```python
from build123d import *
from OCP.BRepFilletAPI import BRepFilletAPI_MakeChamfer

# Parameters (mm, degrees)
SKETCH_1_W               = 23
SKETCH_1_H               = 90
EXTRUDE_1_DEPTH          = 5
SKETCH_2_R               = 4.25
SKETCH_2_R_2             = 6.5
CUT_EXTRUDE_1_DEPTH      = 3.5
EXTRUDE_START            = 15
SKETCH_4_W               = 5
SKETCH_4_H               = 13
EXTRUDE_3_DEPTH          = 30
FILLET_2_R               = 10
CUT_EXTRUDE_2_DEPTH      = 50.812147113
CUT_EXTRUDE_2_DEPTH_BACK = 50.812147113
SKETCH_5_R               = 1.75
FILLET_3_R               = 2.5
EXTRUDE_START_2          = 6.5
EXTRUDE_4_DEPTH          = 5
CHAMFER_1_SIZE           = 1.2
CHAMFER_1_SIZE2          = 0.692820323
FILLET_4_R               = 3


with BuildPart() as part:
    # 스케치1 → 보스-돌출1 (new, symmetric)
    with BuildSketch(Plane(origin=(0, 0, 0), x_dir=(1, 0, 0), z_dir=(0, 1, 0))):
        Rectangle(SKETCH_1_W, SKETCH_1_H)
    extrude(amount=EXTRUDE_1_DEPTH, both=True)

    # 스케치2 → 컷-돌출1 (cut)
    with BuildSketch(Plane.XZ.offset(5)):
        with Locations((0, 24.25)):
            Circle(SKETCH_2_R)
        with BuildLine():
            ThreePointArc((4.25, 24.25), (-0.19737792, 20.004585773), (-4.231666803, 24.644329897))
            Line((-4.231666803, 24.644329897), (-6.471960993, 0.603092784))
            ThreePointArc((-6.471960993, 0.603092784), (0, 6.5), (6.471960993, 0.603092784))
            Line((6.471960993, 0.603092784), (4.231666803, 24.644329897))
            ThreePointArc((4.231666803, 24.644329897), (4.245414227, 24.44737792), (4.25, 24.25))
        make_face()
        Circle(SKETCH_2_R_2)
        with BuildLine():
            ThreePointArc((6.471960993, -0.603092784), (0, -6.5), (-6.471960993, -0.603092784))
            Line((-6.471960993, -0.603092784), (-4.231666803, -24.644329897))
            ThreePointArc((-4.231666803, -24.644329897), (-0.19737792, -20.004585773), (4.25, -24.25))
            ThreePointArc((4.25, -24.25), (4.245414227, -24.44737792), (4.231666803, -24.644329897))
            Line((4.231666803, -24.644329897), (6.471960993, -0.603092784))
        make_face()
        with Locations((0, -24.25)):
            Circle(SKETCH_2_R)
    extrude(amount=-CUT_EXTRUDE_1_DEPTH, mode=Mode.SUBTRACT)

    # 스케치4 → 보스-돌출3 (add)
    with BuildSketch(Plane.XY.offset(EXTRUDE_START)):
        with Locations((-9, 11.5)):
            Rectangle(SKETCH_4_W, SKETCH_4_H)
        with Locations((9, 11.5)):
            Rectangle(SKETCH_4_W, SKETCH_4_H)
    extrude(amount=EXTRUDE_3_DEPTH)

    # 필렛2
    fillet_2_edges = [part.edges().sort_by_distance(p)[0] for p in [
        (-11.5, 0, -45),
        (11.5, 0, -45),
    ]]
    fillet(fillet_2_edges, radius=FILLET_2_R)

    # 스케치5 → 컷-돌출2 (cut, two sides: drawn at the far end of the back side and taken through both)
    with BuildSketch(Plane(origin=(0, 0, 0), x_dir=(0, 0, -1), z_dir=(1, 0, 0)).offset(-CUT_EXTRUDE_2_DEPTH_BACK)):
        with Locations((-22.5, 11.5)):
            Circle(SKETCH_5_R)
        with Locations((-37.5, 11.5)):
            Circle(SKETCH_5_R)
    extrude(amount=CUT_EXTRUDE_2_DEPTH + CUT_EXTRUDE_2_DEPTH_BACK, mode=Mode.SUBTRACT)

    # 필렛3
    fillet_3_edges = [part.edges().sort_by_distance(p)[0] for p in [
        (11.5, 6.5, 45),
        (-11.5, 6.5, 45),
    ]]
    fillet(fillet_3_edges, radius=FILLET_3_R)

    # 스케치6 → 보스-돌출4 (add)
    with BuildSketch(Plane(origin=(0, 0, 0), x_dir=(0, 0, -1), z_dir=(1, 0, 0)).offset(EXTRUDE_START_2)):
        Polygon((-15, 18), (25, 5), (-15, 5), align=None)
    extrude_4 = extrude(amount=EXTRUDE_4_DEPTH)

    # 대칭 복사1: 보스-돌출4 across plane
    add(extrude_4.mirror(Plane(origin=(0, 0, 0), x_dir=(0, 0, 1), z_dir=(1, 0, 0))))

    # 모따기1: one chamfer whose edges measure the first distance from different faces: ONE call of the kernel's chamfer builder (chamfer() names one face for all edges)
    chamfer_1_edges_1 = [part.edges().sort_by_distance(p)[0] for p in [
        (5.351813898, -5, 12.62371134),
    ]]
    chamfer_1_side_1 = [part.faces().sort_by_distance(p)[0] for p in [
        (5.351813898, -3.25, 12.62371134),
    ]]
    chamfer_1_edges_2 = [part.edges().sort_by_distance(p)[0] for p in [
        (5.351813898, -5, -12.62371134),
    ]]
    chamfer_1_side_2 = [part.faces().sort_by_distance(p)[0] for p in [
        (5.351813898, -3.25, -12.62371134),
    ]]
    chamfer_1_edges_3 = [part.edges().sort_by_distance(p)[0] for p in [
        (0, -5, 28.5),
    ]]
    chamfer_1_side_3 = [part.faces().sort_by_distance(p)[0] for p in [
        (0, -3.25, 28.5),
    ]]
    chamfer_1_edges_4 = [part.edges().sort_by_distance(p)[0] for p in [
        (-5.351813898, -5, 12.62371134),
    ]]
    chamfer_1_side_4 = [part.faces().sort_by_distance(p)[0] for p in [
        (-5.351813898, -3.25, 12.62371134),
    ]]
    chamfer_1_edges_5 = [part.edges().sort_by_distance(p)[0] for p in [
        (-6.5, -5, 0),
    ]]
    chamfer_1_side_5 = [part.faces().sort_by_distance(p)[0] for p in [
        (-6.5, -3.25, 0),
    ]]
    chamfer_1_edges_6 = [part.edges().sort_by_distance(p)[0] for p in [
        (-5.351813898, -5, -12.62371134),
    ]]
    chamfer_1_side_6 = [part.faces().sort_by_distance(p)[0] for p in [
        (-5.351813898, -3.25, -12.62371134),
    ]]
    chamfer_1_edges_7 = [part.edges().sort_by_distance(p)[0] for p in [
        (0, -5, -28.5),
    ]]
    chamfer_1_side_7 = [part.faces().sort_by_distance(p)[0] for p in [
        (0, -3.25, -28.5),
    ]]
    chamfer_1_edges_8 = [part.edges().sort_by_distance(p)[0] for p in [
        (6.5, -5, 0),
    ]]
    chamfer_1_side_8 = [part.faces().sort_by_distance(p)[0] for p in [
        (6.5, -3.25, 0),
    ]]
    chamfer_1_edges_9 = [part.edges().sort_by_distance(p)[0] for p in [
        (0, -5, -45),
    ]]
    chamfer_1_side_9 = [part.faces().sort_by_distance(p)[0] for p in [
        (0, 0, -45),
    ]]
    chamfer_1_edges_10 = [part.edges().sort_by_distance(p)[0] for p in [
        (-11.5, -5, 3.75),
    ]]
    chamfer_1_side_10 = [part.faces().sort_by_distance(p)[0] for p in [
        (-11.5, 4.599741569, 9.495989177),
    ]]
    chamfer_1_edges_11 = [part.edges().sort_by_distance(p)[0] for p in [
        (-8.571067812, -5, -42.071067812),
    ]]
    chamfer_1_side_11 = [part.faces().sort_by_distance(p)[0] for p in [
        (-8.571067812, 0, -42.071067812),
    ]]
    chamfer_1_edges_12 = [part.edges().sort_by_distance(p)[0] for p in [
        (8.571067812, -5, -42.071067812),
    ]]
    chamfer_1_side_12 = [part.faces().sort_by_distance(p)[0] for p in [
        (8.571067812, 0, -42.071067812),
    ]]
    chamfer_1_edges_13 = [part.edges().sort_by_distance(p)[0] for p in [
        (0, -5, 45),
    ]]
    chamfer_1_side_13 = [part.faces().sort_by_distance(p)[0] for p in [
        (0, 3.051020408, 45),
    ]]
    chamfer_1_edges_14 = [part.edges().sort_by_distance(p)[0] for p in [
        (11.5, -5, 3.75),
    ]]
    chamfer_1_side_14 = [part.faces().sort_by_distance(p)[0] for p in [
        (11.5, 4.599741569, 9.495989177),
    ]]
    chamfer_1_edges_15 = [part.edges().sort_by_distance(p)[0] for p in [
        (10.767766953, -5, 44.267766953),
    ]]
    chamfer_1_side_15 = [part.faces().sort_by_distance(p)[0] for p in [
        (10.767766953, 6.5, 44.267766953),
    ]]
    chamfer_1_edges_16 = [part.edges().sort_by_distance(p)[0] for p in [
        (-10.767766953, -5, 44.267766953),
    ]]
    chamfer_1_side_16 = [part.faces().sort_by_distance(p)[0] for p in [
        (-10.767766953, 6.5, 44.267766953),
    ]]
    chamfer_1 = BRepFilletAPI_MakeChamfer(part.part.solid().wrapped)
    for e in chamfer_1_edges_1:
        chamfer_1.Add(CHAMFER_1_SIZE, CHAMFER_1_SIZE2, e.wrapped, chamfer_1_side_1[0].wrapped)  # the first distance lies on this face
    for e in chamfer_1_edges_2:
        chamfer_1.Add(CHAMFER_1_SIZE, CHAMFER_1_SIZE2, e.wrapped, chamfer_1_side_2[0].wrapped)  # the first distance lies on this face
    for e in chamfer_1_edges_3:
        chamfer_1.Add(CHAMFER_1_SIZE, CHAMFER_1_SIZE2, e.wrapped, chamfer_1_side_3[0].wrapped)  # the first distance lies on this face
    for e in chamfer_1_edges_4:
        chamfer_1.Add(CHAMFER_1_SIZE, CHAMFER_1_SIZE2, e.wrapped, chamfer_1_side_4[0].wrapped)  # the first distance lies on this face
    for e in chamfer_1_edges_5:
        chamfer_1.Add(CHAMFER_1_SIZE, CHAMFER_1_SIZE2, e.wrapped, chamfer_1_side_5[0].wrapped)  # the first distance lies on this face
    for e in chamfer_1_edges_6:
        chamfer_1.Add(CHAMFER_1_SIZE, CHAMFER_1_SIZE2, e.wrapped, chamfer_1_side_6[0].wrapped)  # the first distance lies on this face
    for e in chamfer_1_edges_7:
        chamfer_1.Add(CHAMFER_1_SIZE, CHAMFER_1_SIZE2, e.wrapped, chamfer_1_side_7[0].wrapped)  # the first distance lies on this face
    for e in chamfer_1_edges_8:
        chamfer_1.Add(CHAMFER_1_SIZE, CHAMFER_1_SIZE2, e.wrapped, chamfer_1_side_8[0].wrapped)  # the first distance lies on this face
    for e in chamfer_1_edges_9:
        chamfer_1.Add(CHAMFER_1_SIZE, CHAMFER_1_SIZE2, e.wrapped, chamfer_1_side_9[0].wrapped)  # the first distance lies on this face
    for e in chamfer_1_edges_10:
        chamfer_1.Add(CHAMFER_1_SIZE, CHAMFER_1_SIZE2, e.wrapped, chamfer_1_side_10[0].wrapped)  # the first distance lies on this face
    for e in chamfer_1_edges_11:
        chamfer_1.Add(CHAMFER_1_SIZE, CHAMFER_1_SIZE2, e.wrapped, chamfer_1_side_11[0].wrapped)  # the first distance lies on this face
    for e in chamfer_1_edges_12:
        chamfer_1.Add(CHAMFER_1_SIZE, CHAMFER_1_SIZE2, e.wrapped, chamfer_1_side_12[0].wrapped)  # the first distance lies on this face
    for e in chamfer_1_edges_13:
        chamfer_1.Add(CHAMFER_1_SIZE, CHAMFER_1_SIZE2, e.wrapped, chamfer_1_side_13[0].wrapped)  # the first distance lies on this face
    for e in chamfer_1_edges_14:
        chamfer_1.Add(CHAMFER_1_SIZE, CHAMFER_1_SIZE2, e.wrapped, chamfer_1_side_14[0].wrapped)  # the first distance lies on this face
    for e in chamfer_1_edges_15:
        chamfer_1.Add(CHAMFER_1_SIZE, CHAMFER_1_SIZE2, e.wrapped, chamfer_1_side_15[0].wrapped)  # the first distance lies on this face
    for e in chamfer_1_edges_16:
        chamfer_1.Add(CHAMFER_1_SIZE, CHAMFER_1_SIZE2, e.wrapped, chamfer_1_side_16[0].wrapped)  # the first distance lies on this face
    add(Compound.cast(chamfer_1.Shape()), mode=Mode.REPLACE)

    # 필렛4
    fillet_4_edges = [part.edges().sort_by_distance(p)[0] for p in [
        (5.351813898, -3.8, -12.62371134),
        (6.5, -3.8, 0),
        (0, -3.8, -28.5),
        (5.351813898, -3.8, 12.62371134),
        (-5.351813898, -3.8, -12.62371134),
        (0, -3.8, 28.5),
        (-6.5, -3.8, 0),
        (-5.351813898, -3.8, 12.62371134),
        (-11.5, -3.8, 3.75),
        (-10.767766953, -3.8, 44.267766953),
        (-8.571067812, -3.8, -42.071067812),
        (0, -3.8, 45),
        (0, -3.8, -45),
        (10.767766953, -3.8, 44.267766953),
        (8.571067812, -3.8, -42.071067812),
        (11.5, -3.8, 3.75),
    ]]
    fillet(fillet_4_edges, radius=FILLET_4_R)


solid = part.part
```
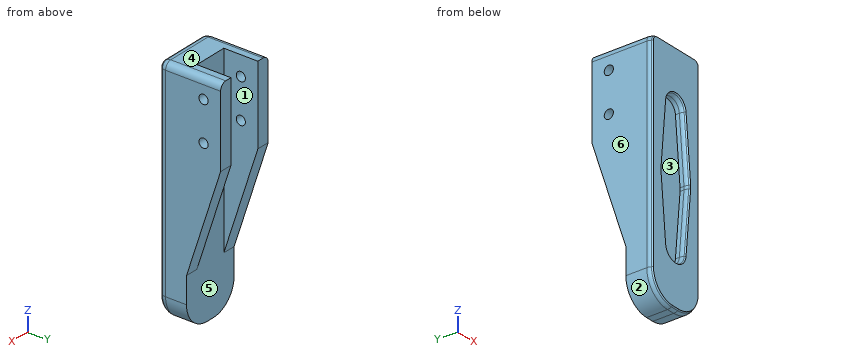
Input: part model. Units: mm. Frame: model coordinates. Face numbers are marked on the shaded views. A direction names the side the tool comes from. Round coordinates to 2 decimals unless told otherwise and drop trailing zeros. Order: outer loops, then holes, each group sorted by start corner. A loop starts at its lowest first (then second) coordinate and runs counter-clockwise, first axis right, second up. Notation, with made-up numbers: (-20.5, 9.25) - (6.5, 9.25) arc R12 ccw to (6.5, 15.25) - close; hole circle Ø1 at (-30, -15). An arc over 180 degrees is marked (long way). Answer in a Markdown table with one row per item.
Item 1: Reachability of the marked faces 1 and 2 from +Z, -Z, +X, -X, +Y, -Y: full face, straight path, thin tool, end or side. Return the list, or none.
Model answer:
| item | result |
|---|---|
| face 1 | +Z, -Z, +Y |
| face 2 | -Z, -X, +Y, -Y |
Item 2: Section query B-B (z = 37.5). Return the cut outline in (x, y).
Model answer:
| item | result |
|---|---|
| outline | (-11.5, -3) arc R3 ccw to (-11.1, -4.5) - (-10.81, -5) - (10.81, -5) - (11.1, -4.5) arc R3 ccw to (11.5, -3) - (11.5, 9.75) - (6.5, 9.75) - (6.5, 5) - (-6.5, 5) - (-6.5, 9.75) - (-11.5, 9.75) - close; (-11.5, 13.25) - (-6.5, 13.25) - (-6.5, 18) - (-11.5, 18) - close; (6.5, 13.25) - (11.5, 13.25) - (11.5, 18) - (6.5, 18) - close |
Item 3: Mould query, pull axis X, two halves, no side actions, for the marked faces 3, 4, 5 and 6. Classes: released by +X, released by -X, zero draft, split by the parting line, or undercut.
Model answer:
| item | result |
|---|---|
| face 3 | undercut |
| face 4 | zero draft |
| face 5 | undercut |
| face 6 | released by -X |
Item 4: Line query: line 1 (X direction, y = 11, z = 17.5); line 2 (Y direction, x = 10.5, z = 37.5); line 3 (Y direction, x = -6.25, z = 39). Output: solid intervals per line, ascending.
Model answer:
| item | result |
|---|---|
| line 1 | x = -11.5 to -6.5, 6.5 to 11.5 |
| line 2 | y = -5 to 9.75, 13.25 to 18 |
| line 3 | y = -5 to 5 |
Item 5: Section query C-C (y = 15). Return the cut outline in (x, z).
Model answer:
| item | result |
|---|---|
| outline | (-11.5, 5.77) - (-6.5, 5.77) - (-6.5, 45) - (-9, 45) arc R2.5 ccw to (-11.5, 42.5) - close; (6.5, 5.77) - (11.5, 5.77) - (11.5, 42.5) arc R2.5 ccw to (9, 45) - (6.5, 45) - close |
Item 6: Section query A-A (y = 11.5). Return the cut outline in (x, z), then the cut area to 3 significant figures.
Model answer:
| item | result |
|---|---|
| outline | (-11.5, -5) - (-6.5, -5) - (-6.5, 20.75) - (-11.5, 20.75) - close; (-11.5, 24.25) - (-6.5, 24.25) - (-6.5, 35.75) - (-11.5, 35.75) - close; (-11.5, 39.25) - (-6.5, 39.25) - (-6.5, 45) - (-9, 45) arc R2.5 ccw to (-11.5, 42.5) - close; (6.5, -5) - (11.5, -5) - (11.5, 20.75) - (6.5, 20.75) - close; (6.5, 24.25) - (11.5, 24.25) - (11.5, 35.75) - (6.5, 35.75) - close; (6.5, 39.25) - (11.5, 39.25) - (11.5, 42.5) arc R2.5 ccw to (9, 45) - (6.5, 45) - close |
| area | 427 mm² |
Item 7: Section query D-D (y = 3). Return the cut outline in (x, z), then the cut area to 3 significant figures.
Model answer:
| item | result |
|---|---|
| outline | (-11.5, -35) arc R10 ccw to (-1.5, -45) - (1.5, -45) arc R10 ccw to (11.5, -35) - (11.5, 42.5) arc R2.5 ccw to (9, 45) - (-9, 45) arc R2.5 ccw to (-11.5, 42.5) - close |
| area | 2,020 mm² |
Item 8: Pin query (flat end, axial travel): pin 1 (2 mm diameter, centred on x = 4.5, y = 14, fed in from +Z) (1 decimal); pin 2 (7 mm diameter, centred on x = 0.5, z = -1.5, fed in from +Y); pin 3 (6 mm diameter, centred on x = -5.5, y = -2, fed in from -Z). Return the tip coordinate at first contact, or that it passes through.
Model answer:
| item | result |
|---|---|
| pin 1 | passes through |
| pin 2 | stops at y = 5 |
| pin 3 | stops at z = -44.95 |
